Read the model definition and answer for the solid it produces. Units are mm, in the model's axes. Coordinates: 2 decimals unless noted, no trailing zeros. Write each loop counter-clockwise with the first axis right and the second up, starting at its lowest first coordinate (ties: lowest second). Pieces come first, ordered by that corner, then holes. Notation, with made-up numbers: (83, 30.5) - (123, 30.5) arc R25 cw to (123, 43.5) - close; hole circle Ø6 at (-21, 52.25). An arc over 180 degrees is marked (long way). Use a Markdown table: item, result.
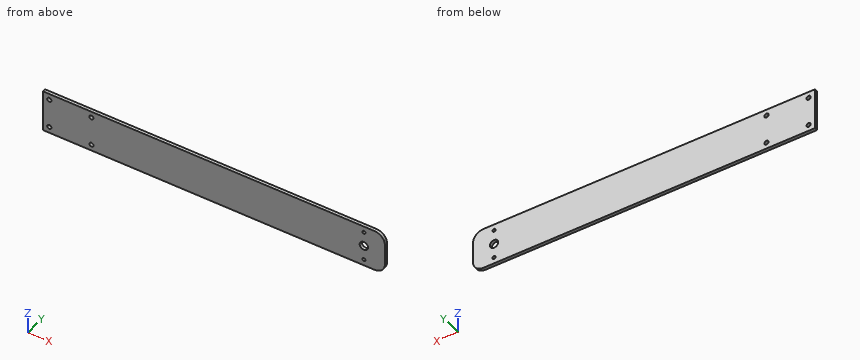
from build123d import *

# Parameters (mm, degrees)
SKETCH1_W           = 325
SKETCH1_H           = 40
SKETCH1_R           = 2
SKETCH1_R_2         = 4
SKETCH1_R_3         = 1.5
BOSS_EXTRUDE1_DEPTH = 3
FILLET1_R           = 10


with BuildPart() as part:
    # Sketch1 → Boss-Extrude1 (new body)
    with BuildSketch(Plane(origin=(0, 0, 0), x_dir=(1, 0, 0), z_dir=(0, 1, 0))):
        Rectangle(SKETCH1_W, SKETCH1_H)
        with Locations(Location((-156.5, 14, 0), (0, 0, 270))):
            Circle(SKETCH1_R, mode=Mode.SUBTRACT)
        with Locations(Location((-116.5, 14, 0), (0, 0, 270))):
            Circle(SKETCH1_R, mode=Mode.SUBTRACT)
        with Locations(Location((-116.5, -14, 0), (0, 0, 270))):
            Circle(SKETCH1_R, mode=Mode.SUBTRACT)
        with Locations(Location((-156.5, -14, 0), (0, 0, 270))):
            Circle(SKETCH1_R, mode=Mode.SUBTRACT)
        with Locations(Location((142.5, 0, 0), (0, 0, 270))):
            Circle(SKETCH1_R_2, mode=Mode.SUBTRACT)
        with Locations(Location((142.5, 14, 0), (0, 0, 270))):
            Circle(SKETCH1_R_3, mode=Mode.SUBTRACT)
        with Locations(Location((142.5, -14, 0), (0, 0, 270))):
            Circle(SKETCH1_R_3, mode=Mode.SUBTRACT)
    extrude(amount=BOSS_EXTRUDE1_DEPTH)

    # Fillet1
    fillet1_edges = [part.edges().sort_by_distance(p)[0] for p in [
        (162.5, 1.5, 20),
        (162.5, 1.5, -20),
    ]]
    fillet(fillet1_edges, radius=FILLET1_R)


solid = part.part
(1) This flat-tipped pin is pushed along its axis until it touches: P1, Ø2.5, axis at x = -116.5, z = 14, coming from the -Y side. Where does it stop, or does it pass through?
Report:
| item | result |
|---|---|
| P1 | passes through |
(2) Straight lines are drawn through the part: L1, parallel to X at y = 1.5, z = -14; L2, parallel to Z at x = -156.5, y = 0.7; L3, parallel to X at y = 2.65, z = 0.5. For each, find the intervals that lie inside material, in ascending order.
Report:
| item | result |
|---|---|
| L1 | x = -162.5 to -158.5, -154.5 to -118.5, -114.5 to 141, 144 to 161.67 |
| L2 | z = -20 to -16, -12 to 12, 16 to 20 |
| L3 | x = -162.5 to 138.53, 146.47 to 162.5 |
(3) A cutting plane is placed at A-A, the plane z = 0. Write down the section's boundary in (x, y), and give its area (3 significant figures).
Report:
| item | result |
|---|---|
| outline | (-162.5, 0) - (138.5, 0) - (138.5, 3) - (-162.5, 3) - close; (146.5, 0) - (162.5, 0) - (162.5, 3) - (146.5, 3) - close |
| area | 951 mm² |
